Geometry: final body of the model. Coordinates: model frame, mm. A direction names the side the tool comes from. Round coordinates to 2 decimals unless told otherwise and drop trailing zeros. Write each loop counter-clockwise with the first axis right and the second up, starting at its lowest first coordinate (ties: lowest second). Pieces come first, ordered by that corner, then holes. Notation, with made-up numbers: M 63,-31.75 L 113,-31.75 A19 cw 113,-0.75 Z; hole C 16,47.25 d10. An arc over 180 degrees is marked long. Use one line per item in the form item = value. Start each with the question number.
Autodesk Fusion 360 part; units mm, degrees
sketch "Sketch1" plane through (0, 0, 0) normal (0, 0, 1) x (1, 0, 0)
  line L0 (45.1, -24.6) -> (-45.1, -24.6)
  line L1 (-45.1, -24.6) -> (-45.1, 24.6)
  line L2 (-45.1, 24.6) -> (45.1, 24.6)
  line L3 (45.1, 24.6) -> (45.1, -24.6)
  line L4 (45.1, -24.6) -> (-45.1, 24.6) construction
  line L5 (-45.1, -24.6) -> (45.1, 24.6) construction
  dimension "d1" = 90.2
  dimension "d2" = 49.2
extrude "Extrude1" add sketch "Sketch1" along normal blind 20
sketch "Sketch2" plane through (0, 0, 0) normal (0, 0, -1) x (-1, 0, 0)
  line L0 (40.1, -22.1) -> (40.1, 22.1)
  line L1 (40.1, 22.1) -> (-40.1, 22.1)
  line L2 (-40.1, 22.1) -> (-40.1, -22.1)
  line L3 (21.6, -24.6) -> (-21.6, -24.6)
  line L4 (-21.6, -24.6) -> (-21.6, 18.6)
  line L5 (-21.6, 18.6) -> (21.6, 18.6)
  line L6 (21.6, 18.6) -> (21.6, -24.6)
  line L7 (45.1, 24.6) -> (-45.1, 24.6)
  line L8 (-45.1, 24.6) -> (-45.1, -24.6)
  line L9 (-45.1, -24.6) -> (45.1, -24.6)
  line L10 (45.1, -24.6) -> (45.1, 24.6)
  dimension "d5" = 43.2
  dimension "d6" = 43.2
  dimension "d73" = 21.6
extrude "Extrude2" cut sketch "Sketch2" against normal blind 11 contours L3 L4 L5 L6 L9
sketch "Sketch3" plane through (0, 24.6, 0) normal (0, 1, 0) x (-1, 0, 0)
  line L0 (-45.1, 0) -> (45.1, 0)
  line L1 (45.1, 0) -> (45.1, 20)
  line L2 (45.1, 20) -> (-45.1, 20)
  line L3 (-45.1, 20) -> (-45.1, 0)
  line L4 (-45.1, 20) -> (-25.1, 20)
  line L5 (-25.1, 20) -> (-25.1, 0)
  line L6 (-25.1, 0) -> (-45.1, 0)
  line L7 (-45.1, 0) -> (-45.1, 20)
  line L8 (45.1, 20) -> (25.1, 20)
  line L9 (25.1, 20) -> (25.1, 0)
  line L10 (25.1, 0) -> (45.1, 0)
  line L11 (45.1, 0) -> (45.1, 20)
  dimension "d9" = 20
  dimension "d10" = 20
extrude "Extrude3" cut sketch "Sketch3" against normal blind 45.2 contours L0 L2 L3 L4 L5 L6 L7 | L0 L1 L2 L8 L9 L10 L11
sketch "Sketch4" plane through (0, 0, 20) normal (0, 0, 1) x (-1, 0, 0)
  line L0 (25.1, -24.6) -> (25.1, 20.6)
  line L1 (25.1, 20.6) -> (45.1, 20.6)
  line L2 (45.1, 20.6) -> (45.1, 24.6)
  line L3 (45.1, 24.6) -> (-45.1, 24.6)
  line L4 (-45.1, 24.6) -> (-45.1, 20.6)
  line L5 (-45.1, 20.6) -> (-25.1, 20.6)
  line L6 (-25.1, 20.6) -> (-25.1, -24.6)
  line L7 (-25.1, -24.6) -> (25.1, -24.6)
  line L8 (25.1, 19) -> (-25.1, 19) construction
  line L9 (25.1, -12) -> (-25.1, -12) construction
  line L10 (15.5, -24.6) -> (15.5, 19) construction
  line L11 (-15.5, -24.6) -> (-15.5, 19) construction
  line L12 (15.5, -12) -> (15.5, -15) construction
  line L13 (15.5, -12) -> (15.5, -15) construction
  line L14 (0, -24.6) -> (0, 24.6) construction
  line L15 (-25.1, 3.5) -> (25.1, 3.5) construction
  circle A0 centre (15.5, -12) radius 1.7
  circle A1 centre (15.5, -12) radius 3
  circle A2 centre (-15.5, -12) radius 1.7
  circle A3 centre (-15.5, -12) radius 3
  circle A4 centre (-15.5, 19) radius 3
  circle A5 centre (-15.5, 19) radius 1.7
  circle A6 centre (15.5, 19) radius 3
  circle A7 centre (15.5, 19) radius 1.7
  dimension "d59" = 9.6
  dimension "d60" = 9.6
  dimension "d68" = 3.4
  dimension "d69" = 6
  dimension "d70" = 31
  dimension "d71" = 15.5
extrude "Extrude5" cut sketch "Sketch4" against normal blind 5 contours A0 | A1 | A2 | A3 | A4 | A5 | A6 | A7
extrude "Extrude4" cut sketch "Sketch4" against normal blind 9 from surface at -5.2 contours A0 | A2 | A5 | A7
sketch "Sketch5" plane through (0, -20.6, 0) normal (0, 1, 0) x (-1, 0, 0)
  line L0 (-45.1, 20) -> (-45.1, 0)
  line L1 (-45.1, 0) -> (-25.1, 0)
  line L2 (-25.1, 0) -> (-25.1, 20)
  line L3 (-25.1, 20) -> (-45.1, 0) construction
  line L4 (-45.1, 20) -> (-25.1, 0) construction
  circle A0 centre (-35.1, 10) radius 2.5
  circle A1 centre (-35.1, 10) radius 4.5
  line L5 (-25.1, 20) -> (-45.1, 20)
  dimension "d33" = 5
  dimension "d34" = 9
extrude "Extrude8" cut sketch "Sketch5" against normal blind 1 contours A0 | A1
extrude "Extrude7" cut sketch "Sketch5" against normal blind 4 contours A0
sketch "Sketch6" plane through (0, -20.6, 0) normal (0, 1, 0) x (-1, 0, 0)
  line L0 (45.1, 0) -> (45.1, 20)
  line L1 (25.1, 20) -> (25.1, 0)
  line L2 (25.1, 0) -> (45.1, 0)
  line L3 (25.1, 0) -> (45.1, 20) construction
  line L4 (25.1, 20) -> (45.1, 0) construction
  circle A0 centre (35.1, 10) radius 2.5
  circle A1 centre (35.1, 10) radius 4.5
  line L5 (45.1, 20) -> (25.1, 20)
  dimension "d39" = 5
  dimension "d40" = 9
extrude "Extrude10" cut sketch "Sketch6" against normal blind 1 contours A0 | A1
extrude "Extrude9" cut sketch "Sketch6" against normal blind 4 contours A0
sketch "Sketch7" plane through (0, 0, 20) normal (0, 0, 1) x (-1, 0, 0)
  line L0 (25.1, -24.6) -> (25.1, 20.6)
  line L1 (25.1, 20.6) -> (45.1, 20.6)
  line L2 (45.1, 20.6) -> (45.1, 24.6)
  line L3 (45.1, 24.6) -> (-45.1, 24.6)
  line L4 (-45.1, 24.6) -> (-45.1, 20.6)
  line L5 (-45.1, 20.6) -> (-25.1, 20.6)
  line L6 (-25.1, 20.6) -> (-25.1, -24.6)
  line L7 (-25.1, -24.6) -> (25.1, -24.6)
  line L8 (-25.1, 0.6) -> (25.1, 0.6) construction
  line L9 (45.1, 24.6) -> (-45.1, 24.6) construction
  line L10 (45.1, 20.6) -> (25.1, 0.6)
  line L11 (-25.1, 0.6) -> (-45.1, 20.6)
  line L12 (15.5, -12) -> (-15.5, 19) construction
  line L13 (15.5, 19) -> (-15.5, -12) construction
  line L14 (25.1, 2) -> (-25.1, 2) construction
  line L15 (-25.1, 0.5) -> (25.1, 0.5) construction
  line L16 (25.1, 3.5) -> (-25.1, 3.5) construction
  line L17 (0, 3.5) -> (0, 3.5473) construction
  circle A0 centre (15.5, -12) radius 3
  circle A1 centre (-15.5, 19) radius 3
  circle A2 centre (15.5, 19) radius 3
  circle A3 centre (-15.5, -12) radius 3
  circle A4 centre (0, 3.5) radius 11.5
  dimension "d50" = 24
  dimension "d64" = 22.6
  dimension "d65" = 1.5
  dimension "d66" = 1.5
  dimension "d74" = 23
extrude "Extrude13" cut sketch "Sketch7" against normal blind 9 contours A4
extrude "Extrude11" add sketch "Sketch7" against normal blind 4 contours L0 L1 L10 | L5 L6 L11
extrude "Extrude12" add sketch "Sketch7" along normal blind 4 from surface at -20 contours L0 L1 L10 | L5 L6 L11
chamfer "Chamfer1" distance 4 angle 45 2 edges at (21.6, 18.6, 5.5) (-21.6, 18.6, 5.5)
equation "d71 = d70 / 2"
equation "d73 = d5 / 2"
1. Contact query for flat-ended pins moving along their axis: pin 1 (6 mm diameter, centred on y = -3.5, z = 15, fed in from -X); pin 2 (4 mm diameter, centred on x = 15.5, y = 12, fed in from +Z); pin 3 (1.5 mm diameter, centred on y = 16.5, z = 14, fed in from +X). Output: stop coordinate, or through.
2. Set-up query: faces 1 (the face through (16, 12, 15)), 2 (the face through (-15, -19, 14.8)), 3 (the face through (31, -15, 16)), 4 (the face through (-33, -13, 4)), 5 (the face through (-37, -21.6, 8)). Return all of +Z, -Z, +X, -X, +Y, -Y with unobstructed straight access to the full face (end or side cutting, diameter ignored); none if empty.
3. Pull-direction query (Y, two-part tool) for faces 6 (the face through (-35.2, -10.7, 18)), 7 (the face through (13.93, 12.65, 12.93)), 8 (the face through (10, -12, 11)), 9 (the face through (-17.07, 12.65, 12.93)); classes: released by +Y, released by -Y, zero draft, split by the parting line, or undercut.
4. Ray query, probe 1 along X at (y, z) = (12, 16.45); probe 2 along X at (y, z) = (12, 12.5); probe 3 along Y at (x, z) = (15.5, 12.7). Return the intervals inside material, ascending.
5. Section query A-A (x = 35.1). Return loops of the section in (y, z), then the cut area to 3 significant figures.
6. Section query D-D (z = 17.75). Return loops of the section in (x, y).
7. Section query B-B (z = 10). Give the number of separate pieces and of enclosed holes in the cut face, then the cut area to 3 significant figures.
8. Section query C-C (y = -3.5). Return loops of the section in (x, z), then the cut area to 3 significant figures.
Checks:
q1.pin_1 = -30.83
q1.pin_2 = 15
q1.pin_3 = 25.1
q2.face_1 = +Z
q2.face_2 = -Z
q2.face_3 = +X, +Y
q2.face_4 = -X, +Y
q2.face_5 = +Y
q3.face_6 = released by +Y
q3.face_7 = undercut
q3.face_8 = zero draft
q3.face_9 = undercut
q4.probe_1 = -25.1 to -18.5, -12.5 to 12.5, 18.5 to 25.1
q4.probe_2 = -25.1 to -17.2, -13.8 to 13.8, 17.2 to 25.1
q4.probe_3 = -24.6 to -20.7, -17.3 to 10.3, 13.7 to 24.6
q5.outline = M -24.6,0 L -10.6,0 L -10.6,4 L -20.6,4 L -20.6,5.5 L -21.6,5.5 L -21.6,7.5 L -24.6,7.5 Z; M -24.6,12.5 L -21.6,12.5 L -21.6,14.5 L -20.6,14.5 L -20.6,16 L -10.6,16 L -10.6,20 L -24.6,20 Z
q5.area = 136 mm^2
q6.outline = M -45.1,-24.6 L 45.1,-24.6 L 45.1,-20.6 L 25.1,-0.6 L 25.1,24.6 L -25.1,24.6 L -25.1,-0.6 L -45.1,-20.6 Z; hole C -15.5,-19 d6; hole C -15.5,12 d6; hole C 0,-3.5 d23; hole C 15.5,-19 d6; hole C 15.5,12 d6
q7.separate_pieces = 3
q7.enclosed_holes = 0
q7.area = 732 mm^2
q8.outline = M -28,0 L -21.6,0 L -21.6,11 L -11.5,11 L -11.5,20 L -28,20 L -28,16 L -25.1,16 L -25.1,4 L -28,4 Z; M 11.5,11 L 21.6,11 L 21.6,0 L 28,0 L 28,4 L 25.1,4 L 25.1,16 L 28,16 L 28,20 L 11.5,20 Z
q8.area = 368 mm^2
